Source: CAD feature listing. Evaluate the final solid. Frame: model axes, mm. A direction names the side the tool comes from. Coordinates: 2 decimals unless noted, no trailing zeros. Order: outer loops, then holes, each group sorted by start corner. A loop starts at its lowest first (then second) coordinate and runs counter-clockwise, first axis right, second up. Notation, with made-up numbers: (28.5, 77.25) -> (38.5, 77.25) arc R31 cw to (38.5, 105.25) -> close; hole circle Ø6 at (72, 85). An arc over 180 degrees is marked (long way). Put each result on its own line as item: value.
from build123d import *

# Parameters (mm, degrees)
F0_R      = 20
F0_R_2    = 12
F1_DEPTH  = 50
F3_R      = 12
F3_R_2    = 7.5
F4_DEPTH  = 37
F6_DEPTH  = 10
F7_DEPTH  = 15
F9_R      = 7.5
F10_DEPTH = 10
F11_W     = 3
F11_H     = 6
F12_DEPTH = 7


with BuildPart() as f1:
    # F0 (on Front) → F1 (new body)
    with BuildSketch(Plane.XZ):
        Circle(F0_R)
        Circle(F0_R_2, mode=Mode.SUBTRACT)
    extrude(amount=F1_DEPTH)

    # F3 (on offset) → F4 (join)
    with BuildSketch(Plane.XZ.offset(13)):
        Circle(F3_R)
        Circle(F3_R_2, mode=Mode.SUBTRACT)
    extrude(amount=F4_DEPTH)

    # F5 (on offset) → F6 (cut)
    with BuildSketch(Plane.XZ.offset(13)):
        with BuildLine():
            ThreePointArc((0.5, 11.9895788083), (0, 12), (-0.5, 11.9895788083))
            Line((-0.5, 11.9895788083), (-0.5, 7.4833147735))
            ThreePointArc((-0.5, 7.4833147735), (0, 7.5), (0.5, 7.4833147735))
            Line((0.5, 7.4833147735), (0.5, 11.9895788083))
        make_face()
    extrude(amount=F6_DEPTH, mode=Mode.SUBTRACT)

    # F5 (on offset) → F7 (cut)
    with BuildSketch(Plane.XZ.offset(13)):
        with BuildLine():
            ThreePointArc((0.5, 11.9895788083), (0, 12), (-0.5, 11.9895788083))
            Line((-0.5, 11.9895788083), (-0.5, 7.4833147735))
            ThreePointArc((-0.5, 7.4833147735), (0, 7.5), (0.5, 7.4833147735))
            Line((0.5, 7.4833147735), (0.5, 11.9895788083))
        make_face()
        with BuildLine():
            ThreePointArc((-6.7307406984, 3.3086446849), (-6.4951905284, 3.75), (-6.2307406984, 4.1746700887))
            Line((-6.2307406984, 4.1746700887), (-10.1332798286, 6.427802106))
            ThreePointArc((-10.1332798286, 6.427802106), (-10.3923048454, 6), (-10.6332798286, 5.5617767022))
            Line((-10.6332798286, 5.5617767022), (-6.7307406984, 3.3086446849))
        make_face()
        with BuildLine():
            ThreePointArc((-6.2307406984, -4.1746700887), (-6.4951905284, -3.75), (-6.7307406984, -3.3086446849))
            Line((-6.7307406984, -3.3086446849), (-10.6332798286, -5.5617767022))
            ThreePointArc((-10.6332798286, -5.5617767022), (-10.3923048454, -6), (-10.1332798286, -6.427802106))
            Line((-10.1332798286, -6.427802106), (-6.2307406984, -4.1746700887))
        make_face()
        with BuildLine():
            ThreePointArc((0.5, -7.4833147735), (0, -7.5), (-0.5, -7.4833147735))
            Line((-0.5, -7.4833147735), (-0.5, -11.9895788083))
            ThreePointArc((-0.5, -11.9895788083), (0, -12), (0.5, -11.9895788083))
            Line((0.5, -11.9895788083), (0.5, -7.4833147735))
        make_face()
        with BuildLine():
            ThreePointArc((6.7307406984, -3.3086446849), (6.4951905284, -3.75), (6.2307406984, -4.1746700887))
            Line((6.2307406984, -4.1746700887), (10.1332798286, -6.427802106))
            ThreePointArc((10.1332798286, -6.427802106), (10.3923048454, -6), (10.6332798286, -5.5617767022))
            Line((10.6332798286, -5.5617767022), (6.7307406984, -3.3086446849))
        make_face()
        with BuildLine():
            ThreePointArc((6.2307406984, 4.1746700887), (6.4951905284, 3.75), (6.7307406984, 3.3086446849))
            Line((6.7307406984, 3.3086446849), (10.6332798286, 5.5617767022))
            ThreePointArc((10.6332798286, 5.5617767022), (10.3923048454, 6), (10.1332798286, 6.427802106))
            Line((10.1332798286, 6.427802106), (6.2307406984, 4.1746700887))
        make_face()
    extrude(amount=F7_DEPTH, mode=Mode.SUBTRACT)

    # F9 (on offset) → F10 (join)
    with BuildSketch(Plane.XZ.offset(50)):
        Circle(F9_R)
    extrude(amount=-F10_DEPTH)

    # F11 (on offset) → F12 (cut)
    with BuildSketch(Plane.XZ.offset(50)):
        Rectangle(F11_W, F11_H)
    extrude(amount=-F12_DEPTH, mode=Mode.SUBTRACT)


solid = f1.part
1. First-contact query: pin 1 (1.4 mm diameter, centred on y = -19.5, z = 9, fed in from -X); pin 2 (2.5 mm diameter, centred on x = -8.5, z = -5.5, fed in from +Y); pin 3 (2 mm diameter, centred on y = -27, z = 10.5, fed in from -X). Flat tips, straight axial feed; report the tip coordinate or a pass-through.
Numbers:
pin 1: stops at x = -18.2
pin 2: stops at y = -13
pin 3: stops at x = -17.6
2. Cut plane B-B on z = 0. Output: boundary loops of the cut face in (x, y), plus the area to 3 significant figures.
Numbers:
outline: (-20, -50) -> (-1.5, -50) -> (-1.5, -43) -> (1.5, -43) -> (1.5, -50) -> (20, -50) -> (20, 0) -> (12, 0) -> (12, -13) -> (7.5, -13) -> (7.5, -40) -> (-7.5, -40) -> (-7.5, -13) -> (-12, -13) -> (-12, 0) -> (-20, 0) -> close
area: 1,260 mm2
3. Cut plane D-D on y = -45.5. Output: boundary loops of the cut face in (x, z), plus the area to 3 significant figures.
Numbers:
outline: circle Ø40 at (0, 0); hole (-1.5, -3) -> (1.5, -3) -> (1.5, 3) -> (-1.5, 3) -> close
area: 1,240 mm2
4. Pull-direction query (Z, two-part tool) for faces 3 (the flat face through (0, -40, 0)), 4 (the flat face through (-8, -28, -5)), 5 (the flat face through (9, 0, -9)); classes: pulls with the +Z half, pulls with the -Z half, needs draft (parallel to the pull), parting line crosses it, or undercut.
Numbers:
face 3: undercut
face 4: undercut
face 5: needs draft
5. Set-up query: faces 1 (the flat face through (-8.655, -20.395, -4.419)), 2 (the flat face through (1.5, -47, 0)). Return all of +Z, -Z, +X, -X, +Y, -Y with unobstructed straight access to the full face (end or side cutting, diameter ignored); none if empty.
Numbers:
face 1: +Y
face 2: -Y
6. Ray query, line 1 along Z through (x, y) = (0, -7); line 2 along Y through (x, z) = (-4.5, 7); line 3 along Z through (x, y) = (1.5, -22). Return the intervals inside material, ascending.
Numbers:
line 1: z = -20 to -12, 12 to 20
line 2: y = -50 to -13
line 3: z = -19.94 to -7.35, 7.35 to 19.94
7. Cut plane A-A on y = -20. Output: boundary loops of the cut face in (x, z), plus the area to 3 significant figures.
Numbers:
outline: circle Ø40 at (0, 0); hole (-10.63, -5.56) arc R12 ccw to (-10.13, -6.43) -> (-6.23, -4.17) arc R7.5 ccw to (-0.5, -7.48) -> (-0.5, -11.99) arc R12 ccw to (0.5, -11.99) -> (0.5, -7.48) arc R7.5 ccw to (6.23, -4.17) -> (10.13, -6.43) arc R12 ccw to (10.63, -5.56) -> (6.73, -3.31) arc R7.5 ccw to (6.73, 3.31) -> (10.63, 5.56) arc R12 ccw to (10.13, 6.43) -> (6.23, 4.17) arc R7.5 ccw to (0.5, 7.48) -> (0.5, 11.99) arc R12 ccw to (-0.5, 11.99) -> (-0.5, 7.48) arc R7.5 ccw to (-6.23, 4.17) -> (-10.13, 6.43) arc R12 ccw to (-10.63, 5.56) -> (-6.73, 3.31) arc R7.5 ccw to (-6.73, -3.31) -> close
area: 1,050 mm2
8. Cut plane C-C on x = 3. Output: boundary loops of the cut face in (y, z).
Numbers:
outline: (-50, -19.77) -> (0, -19.77) -> (0, -11.62) -> (-13, -11.62) -> (-13, -6.87) -> (-40, -6.87) -> (-40, 6.87) -> (-13, 6.87) -> (-13, 11.62) -> (0, 11.62) -> (0, 19.77) -> (-50, 19.77) -> close
